from build123d import *

# Parameters (mm, degrees)
PAD017_DEPTH            = 2
SKETCH057_W             = 70
SKETCH057_H             = 53.34
PAD018_DEPTH            = 40
SKETCH058_W             = 17
SKETCH058_H             = 11.43
SKETCH058_W_2           = 13
SKETCH058_H_2           = 8.89
PAD019_DEPTH            = 11
SKETCH059_R             = 1.5875
POCKET_DEPTH            = 50
BODY012_PLACEMENT_ANGLE = 115


with BuildPart() as part:
    # Sketch056 → Pad017 (new body)
    with BuildSketch(Plane.XY):
        Polygon((-101.6, 53.34), (-2.54, 53.34), (0, 50.8), (0, 40.64), (2.54, 38.1), (2.54, 3.81), (0, 1.27), (0, 0), (-101.6, 0), (-101.6, 3.175), (-103.505, 3.175), (-103.505, 12.065), (-101.6, 12.065), (-101.6, 32.385), (-107.95, 32.385), (-107.95, 43.815), (-101.6, 43.815), align=None)
    extrude(amount=PAD017_DEPTH)

    # Sketch057 (on Face19 of Pad017) → Pad018 (join)
    with BuildSketch(Plane.XY.offset(2)):
        with Locations((-66.6, 26.67)):
            Rectangle(SKETCH057_W, SKETCH057_H)
    extrude(amount=PAD018_DEPTH)

    # Sketch058 (on Face24 of Pad018) → Pad019 (join)
    with BuildSketch(Plane.XY.offset(2)):
        with Locations((-99.45, 38.1)):
            Rectangle(SKETCH058_W, SKETCH058_H)
        with Locations((-97.005, 7.62)):
            Rectangle(SKETCH058_W_2, SKETCH058_H_2)
    extrude(amount=PAD019_DEPTH)

    # Sketch059 (on Face4 of Pad019) → Pocket (cut)
    with BuildSketch(Plane(origin=(0, 0, 0), x_dir=(1, 0, 0), z_dir=(0, 0, -1))):
        with Locations((-86.36, -2.54)):
            Circle(SKETCH059_R)
        with Locations((-11.43, -2.54)):
            Circle(SKETCH059_R)
        with Locations((-87.63, -50.8)):
            Circle(SKETCH059_R)
        with Locations((-5.08, -50.8)):
            Circle(SKETCH059_R)
        with Locations((-35.56, -17.78)):
            Circle(SKETCH059_R)
        with Locations((-35.56, -45.72)):
            Circle(SKETCH059_R)
    extrude(amount=-POCKET_DEPTH, mode=Mode.SUBTRACT)


with BuildPart() as part_1:
    # Body012 placement: moved
    add(part.part.moved(Location((2.7561582663, -32.0302512871, 15.15))).rotate(Axis((2.7561582663, -32.0302512871, 15.15), (0, 0, -1)), BODY012_PLACEMENT_ANGLE))


solid = part_1.part
Check sheet for the modelled part. Datum: model origin and axes. Units: mm. A direction names the side the tool comes from. Give positions to 0.01 mm unless a question says otherwise; leave off trailing zeros. Write each loop counter-clockwise with the first axis right and the second up, starting at its lowest first coordinate (ties: lowest second). Pieces come first, ordered by that corner, then holes. Notation, with made-up numbers: M 28.5,-10 L 81.5,-10 A8 ccw 81.5,2 Z; hole C 11.25,-7 d1. An arc over 180 degrees is marked long. Use one line per item in the form item = value.
(1) Depth check by flat-ended pin: P1, Ø1.5, axis at x = 12, y = -13.5, coming from the +Z side; P2, Ø3.5, axis at x = 41.56, y = 45.17, coming from the -Z side; P3, Ø4, axis at x = 70.5, z = 40, coming from the -Y side; P4, Ø3, axis at y = 30, z = 41.5, coming from the +X side (3 decimals). Enter the tip coordinate at first touch or a pass-through.
Answer block:
P1 = 17.15
P2 = 15.15
P3 = -17.26
P4 = 91.235
(2) Section check C-C on y = -40. Record the boundary of the cut face in (x, z), plus the area to 3 significant figures.
Answer block:
outline = M 13.84,15.15 L 57.89,15.15 L 57.89,17.15 L 13.84,17.15 Z
area = 88.1 mm2
(3) Tool access check on faces 4 (the flat face through (53, 58, 28.15)), 5 (the flat face through (33, -31, 17.15)), 6 (the flat face through (44.257, -51.382, 16.136)). Record the directions out of +Z, -Z, +X, -X, +Y, -Y that give a thin tool (end or side, any length) a straight path to the whole face; none if there is none.
Answer block:
face_4 = +Z, +X, +Y
face_5 = +Z, -X, -Y
face_6 = +Z, -Z, -Y
(4) Draft check along X on faces 1 (the flat face through (69.527, 48.937, 35.856)), 2 (the flat face through (39.944, -14.504, 36.87)), 3 (the flat face through (86.765, 44.451, 21.559)). Enter one of: pulls with the +X half, pulls with the -X half, needs draft (parallel to the pull), parting line crosses it, or undercut.
Answer block:
face_1 = undercut
face_2 = pulls with the -X half
face_3 = pulls with the +X half
(5) Material ranges on line 1 along Z through (x, y) = (35, -15.5); line 2 along X through (y, z) = (-19.5, 53); line 3 along X through (y, z) = (44, 28.5), recorded low to high.
Answer block:
line_1 = 15.15 to 17.15
line_2 = 50.66 to 57.68, 60.76 to 67.45
line_3 = 38.21 to 40.48, 42.63 to 80.11
(6) Section check B-B on x = 20. Record the boundary of the cut face in (y, z), plus the area to 3 significant figures.
Answer block:
outline = M -42.87,15.15 L 4.95,15.15 L 4.95,57.15 L -5.2,57.15 L -5.2,17.15 L -42.87,17.15 Z
area = 502 mm2
(7) Section check A-A on z = 21. Record the boundary of the cut face in (x, y) (1 decimal), plus the area to 3 significant figures.
Answer block:
outline = M 16.1,-3.4 L 64.5,-25.9 L 94,37.5 L 85.4,41.5 L 88.1,47.3 L 77.7,52.1 L 75,46.4 L 56.6,55 L 57.4,56.7 L 49.4,60.4 L 48.6,58.7 L 45.7,60.1 Z; hole C 33.9,-7.3 d3.2; hole C 41.6,45.2 d3.2; hole C 59.2,-19.1 d3.2; hole C 85.8,25.9 d3.2
area = 3,790 mm2
(8) Section check D-D on z = 41. Record the boundary of the cut face in (x, y) (1 decimal), plus the area to 3 significant figures.
Answer block:
outline = M 16.1,-3.4 L 64.5,-25.9 L 94,37.5 L 45.7,60.1 Z; hole C 33.9,-7.3 d3.2; hole C 41.6,45.2 d3.2; hole C 59.2,-19.1 d3.2; hole C 85.8,25.9 d3.2
area = 3,700 mm2
